from build123d import *

# Parameters (mm, degrees)
SKETCH_1_R      = 1.6
SKETCH_1_R_2    = 1.7
SKETCH_1_R_3    = 20
EXTRUDE_1_DEPTH = 3


with BuildPart() as part:
    # 草图1 → 凸台-拉伸1 (new body)
    with BuildSketch(Plane.XY):
        with BuildLine():
            Line((21, 58), (-21, 58))
            ThreePointArc((-21, 58), (-24.190987584, 56.849363355), (-25.913308269, 53.927039296))
            Line((-25.913308269, 53.927039296), (-35.913308269, 0.927039296))
            ThreePointArc((-35.913308269, 0.927039296), (-35.679941102, -1.760156608), (-34.084620834, -3.935112998))
            Line((-34.084620834, -3.935112998), (-3.084620834, -28.235112998))
            ThreePointArc((-3.084620834, -28.235112998), (0, -29.3), (3.084620834, -28.235112998))
            Line((3.084620834, -28.235112998), (34.084620834, -3.935112998))
            ThreePointArc((34.084620834, -3.935112998), (35.679941102, -1.760156608), (35.913308269, 0.927039296))
            Line((35.913308269, 0.927039296), (25.913308269, 53.927039296))
            ThreePointArc((25.913308269, 53.927039296), (24.190987584, 56.849363355), (21, 58))
        make_face()
        with Locations((21, 53)):
            Circle(SKETCH_1_R, mode=Mode.SUBTRACT)
        with Locations((-21, 53)):
            Circle(SKETCH_1_R, mode=Mode.SUBTRACT)
        with Locations((31, 0)):
            Circle(SKETCH_1_R_2, mode=Mode.SUBTRACT)
        with Locations((-31, 0)):
            Circle(SKETCH_1_R_2, mode=Mode.SUBTRACT)
        with Locations((18, 47)):
            Circle(SKETCH_1_R, mode=Mode.SUBTRACT)
        with Locations((-18, 47)):
            Circle(SKETCH_1_R, mode=Mode.SUBTRACT)
        with Locations((0, -24.3)):
            Circle(SKETCH_1_R, mode=Mode.SUBTRACT)
        with Locations((0, 20)):
            Circle(SKETCH_1_R_3, mode=Mode.SUBTRACT)
    extrude(amount=EXTRUDE_1_DEPTH)


solid = part.part
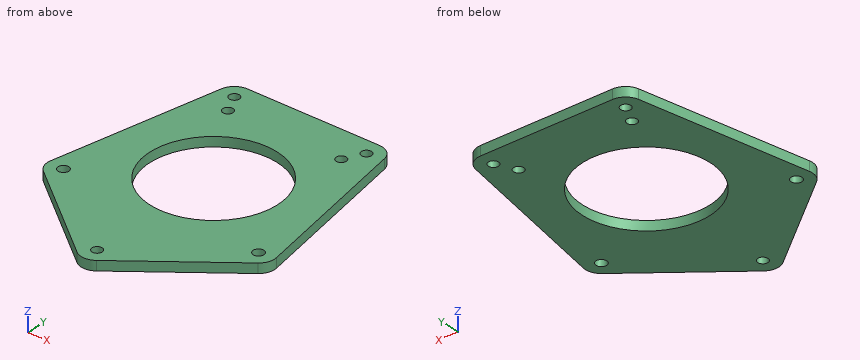
Could you check a few things on this model? Use its own coordinates, in mm. Coordinates: 2 decimals unless noted, no trailing zeros. Write each loop counter-clockwise with the first axis right and the second up, starting at its lowest first coordinate (ties: lowest second). Pieces come first, ordered by that corner, then holes. Notation, with made-up numbers: (-35, 86) - (17, 86) arc R22 cw to (17, 101) - close; hole circle Ø11 at (4.5, 59). An arc over 180 degrees is marked (long way). Put each result on its own line as item: value. Start each with the question number.
Q1. I want a section at C-C on z = 1.4. Count the separate pieces of the cut face and the enclosed holes in it, plus the area to 3 significant figures.
Q2. Please list where these lines run through material, in increasing order: L1, parallel to Y at x = 18, z = 2.35; L2, parallel to X at y = 47.5, z = 1.8; L3, parallel to Y at x = 15, z = 0.45 (3 decimals).
Q3. I want a section at D-D on x = -10.5. Write out the boundary of the cut face in (y, z).
Q4. I'm going to push flat-ended pins straight in: P1, Ø2.5, axis at x = 21, y = 53, coming from the +Z side; P2, Ø1, axis at y = 45.5, z = 0.5, coming from the +X side; P3, Ø1.5, axis at y = 40.5, z = 1.5, coming from the +X side; P4, Ø1.5, axis at y = 39, z = 1.5, coming from the -X side. Where does each tip first touch, or does it pass through?
Q5. I want a section at A-A on x = 0. Write out the boundary of the cut face in (y, z).
Q6. I want a section at B-B on y = 7.5. Write out the boundary of the cut face in (x, z).
Checks:
1. separate pieces: 1
1. enclosed holes: 8
1. area: 3,420 mm²
2. L1: -16.54 to 11.28, 28.72 to 45.4, 48.6 to 58
2. L2: -27.13 to -19.52, -16.48 to 16.48, 19.52 to 27.13
2. L3: -18.895 to 6.771, 33.229 to 58
3. outline: (-22.42, 0) - (2.98, 0) - (2.98, 3) - (-22.42, 3) - close; (37.02, 0) - (58, 0) - (58, 3) - (37.02, 3) - close
4. P1: through
4. P2: x = 27.6
4. P3: x = 28.59
4. P4: x = -28.87
5. outline: (-29.3, 0) - (-25.9, 0) - (-25.9, 3) - (-29.3, 3) - close; (-22.7, 0) - (0, 0) - (0, 3) - (-22.7, 3) - close; (40, 0) - (58, 0) - (58, 3) - (40, 3) - close
6. outline: (-34.67, 0) - (-15.61, 0) - (-15.61, 3) - (-34.67, 3) - close; (15.61, 0) - (34.67, 0) - (34.67, 3) - (15.61, 3) - close
